Verification items for the finished model (mm, model axes). A direction names the side the tool comes from. Coordinates: 2 decimals unless noted, no trailing zeros. Order: outer loops, then holes, each group sorted by start corner. A loop starts at its lowest first (then second) coordinate and runs counter-clockwise, first axis right, second up. Notation, with made-up numbers: (17, 14.5) -> (68, 14.5) arc R24 cw to (68, 42.5) -> close; hole circle Ø6 at (36, 27). An arc over 180 degrees is marked (long way). Write item = value, one per line. Start each with the question number.
1. Cross-section at A-A on x = 83. Record the cut outline in (y, z), plus the area to 3 significant figures.
2. Thickness scan on line 1 along Y through (x, z) = (78, 8.25); line 2 along X through (y, z) = (-8.5, 27); line 3 along Z through (x, y) = (26.5, -33). Record the ranges inside material, lowest first. Write a range as from..to.
3. Set-up check for faces 4 (the flat face through (93, -5, 30)), 5 (the flat face through (93, -10, 25)), 6 (the flat face through (5, -30, 30)), 7 (the flat face through (88, -5, 25)): record each of +Z, -Z, +X, -X, +Y, -Y from which the full face is reachable in a straight line by a thin tool's end or side.
4. Cross-section at C-C on x = 8.5. Record the cut outline in (y, z), plus the area to 3 significant figures.
5. Cross-section at D-D on z = 38.5. Record the cut outline in (x, y).
6. Go/stop test with flat-tipped pins: P1, Ø10, axis at y = -30, z = 27.5, coming from the +X side; P2, Ø15.5, axis at x = 65.5, y = -37, coming from the +Z side; P3, Ø3, axis at x = 7.5, y = -34, coming from the +Z side. Record where each tip stops, or that it passes through.
7. Release check for a two-part mould opening along X. For faces 1 (the flat face through (15, -10, 28)), 2 (the flat face through (20, -5, 25)), 3 (the flat face through (98, -16, 11)) record: +X half, -X half, draft (parallel to the pull), parting line (faces both ways), or undercut.
8. Cross-section at B-B on y = -7. Record the cut outline in (x, z), plus the area to 3 significant figures.
from build123d import *

# Parameters (mm, degrees)
SKETCH2_W               = 10
SKETCH2_H               = 10
BOSS_EXTRUDE2_DEPTH     = 30
SKETCH2_5_R             = 10
BOSS_EXTRUDE3_DEPTH     = 20
SKETCH2_6_W             = 10
SKETCH2_6_H             = 10
BOSS_EXTRUDE4_DEPTH     = 40
SKETCH2_7_W             = 10
SKETCH2_7_H             = 21
BOSS_EXTRUDE5_DEPTH     = 30
SKETCH2_8_W             = 10
SKETCH2_8_H             = 10
BOSS_EXTRUDE6_DEPTH     = 40
SKETCH2_9_W             = 10
SKETCH2_9_H             = 10
BOSS_EXTRUDE7_DEPTH     = 30
SKETCH2_10_W            = 10
SKETCH2_10_H            = 10
BOSS_EXTRUDE8_DEPTH     = 40
CUT_EXTRUDE3_DEPTH      = 114.512113891
CUT_EXTRUDE3_DEPTH_BACK = 10
CUT_EXTRUDE5_START      = -10
CUT_EXTRUDE5_DEPTH      = 10
CUT_EXTRUDE6_DEPTH      = 110.293183685
CUT_EXTRUDE6_DEPTH_BACK = 10


# Read off the part's stored shape, not the designer's step: Cut-Extrude5
with BuildPart() as part:
    # Sketch2 → Boss-Extrude2 (new body)
    with BuildSketch(Plane.XY):
        with Locations((93, -5)):
            Rectangle(SKETCH2_W, SKETCH2_H)
    extrude(amount=BOSS_EXTRUDE2_DEPTH)

    # Sketch2<5> → Boss-Extrude3 (add)
    with BuildSketch(Plane.XY):
        with BuildLine():
            Line((88, 0), (20, 0))
            Line((20, 0), (20, -10))
            Line((20, -10), (10, -10))
            Line((10, -10), (10, -20))
            Line((10, -20), (10, -41))
            Line((10, -41), (10, -51))
            Line((10, -51), (78, -51))
            ThreePointArc((78, -51), (92.142135624, -45.142135624), (98, -31))
            Line((98, -31), (98, -10))
            Line((98, -10), (88, -10))
            Line((88, -10), (88, 0))
        make_face()
        with Locations((78, -31)):
            Circle(SKETCH2_5_R, mode=Mode.SUBTRACT)
    extrude(amount=BOSS_EXTRUDE3_DEPTH)

    # Sketch2<7> → Boss-Extrude5 (add)
    with BuildSketch(Plane.XY):
        with Locations((5, -30.5)):
            Rectangle(SKETCH2_7_W, SKETCH2_7_H)
    extrude(amount=BOSS_EXTRUDE5_DEPTH)



with BuildPart() as body_2:
    # Sketch2<6> → Boss-Extrude4 (new body)
    with BuildSketch(Plane.XY):
        with Locations((5, -5)):
            Rectangle(SKETCH2_6_W, SKETCH2_6_H)
    extrude(amount=BOSS_EXTRUDE4_DEPTH)


with BuildPart() as part_1:
    add(part.part)

    add(body_2.part)  # Boss-Extrude6 merges body 2
    # Sketch2<8> → Boss-Extrude6 (add)
    with BuildSketch(Plane.XY):
        with Locations((15, -5)):
            Rectangle(SKETCH2_8_W, SKETCH2_8_H)
    extrude(amount=BOSS_EXTRUDE6_DEPTH)

    # Sketch2<9> → Boss-Extrude7 (add)
    with BuildSketch(Plane.XY):
        with Locations((5, -46)):
            Rectangle(SKETCH2_9_W, SKETCH2_9_H)
    extrude(amount=BOSS_EXTRUDE7_DEPTH)

    # Sketch2<10> → Boss-Extrude8 (add)
    with BuildSketch(Plane.XY):
        with Locations((5, -15)):
            Rectangle(SKETCH2_10_W, SKETCH2_10_H)
    extrude(amount=BOSS_EXTRUDE8_DEPTH)

    # Sketch6 → Cut-Extrude3 (cut, two sides: drawn at the far end of the back side and taken through both)
    with BuildSketch(Plane.XZ.offset(10).offset(-CUT_EXTRUDE3_DEPTH_BACK)):
        Polygon((20, 40), (10, 40), (20, 30), align=None)
    extrude(amount=CUT_EXTRUDE3_DEPTH + CUT_EXTRUDE3_DEPTH_BACK, mode=Mode.SUBTRACT)

    # Cut-Extrude5 outline → Cut-Extrude5 (cut)
    with BuildSketch(Plane(origin=(10, 0, 0), x_dir=(0, 0, -1), z_dir=(1, 0, 0)).offset(CUT_EXTRUDE5_START)):
        Polygon((-40, -20), (-30, -20), (-40, -10), align=None)
    extrude(amount=CUT_EXTRUDE5_DEPTH, mode=Mode.SUBTRACT)

    # Sketch8 → Cut-Extrude6 (cut, two sides: drawn at the far end of the back side and taken through both)
    with BuildSketch(Plane(origin=(10, 0, 0), x_dir=(0, 0, -1), z_dir=(1, 0, 0)).offset(-CUT_EXTRUDE6_DEPTH_BACK)):
        Polygon((64.543643605, -135.543643605), (-20, -51), (-30, -41), (-114.543643605, 43.543643605), (-283.630930815, -125.543643605), (-104.543643605, -304.630930815), align=None)
    extrude(amount=CUT_EXTRUDE6_DEPTH + CUT_EXTRUDE6_DEPTH_BACK, mode=Mode.SUBTRACT)


solid = part_1.part
Worked out:
q1.outline = (-50.36, 0) -> (-39.66, 0) -> (-39.66, 20) -> (-50.36, 20) -> close; (-22.34, 0) -> (0, 0) -> (0, 20) -> (-22.34, 20) -> close
q1.area = 661 mm²
q2.line_1 = -51..-41, -21..0
q2.line_2 = 0..20, 88..98
q2.line_3 = 0..20
q3.face_4 = +Z, +X, +Y, -Y
q3.face_5 = +Z, +X, -Y
q3.face_6 = +Z, +X, -X, -Y
q3.face_7 = +Z, +Y, -Y
q4.outline = (-51, 0) -> (0, 0) -> (0, 40) -> (-10, 40) -> (-20, 30) -> (-41, 30) -> (-51, 20) -> close
q4.area = 1,630 mm²
q5.outline = (0, -11.5) -> (10, -11.5) -> (10, -10) -> (11.5, -10) -> (11.5, 0) -> (0, 0) -> close
q6.P1 = 10
q6.P2 = 20
q6.P3 = 30
q7.face_1 = draft
q7.face_2 = undercut
q7.face_3 = +X half
q8.outline = (0, 0) -> (98, 0) -> (98, 30) -> (88, 30) -> (88, 20) -> (20, 20) -> (20, 30) -> (10, 40) -> (0, 40) -> close
q8.area = 2,410 mm²
